Here's how the part is built. I have some questions about the finished solid (model axes, mm). Face numbers are marked on the shaded views. A direction names the side the tool comes from. Coordinates: 2 decimals unless noted, no trailing zeros. Write each loop counter-clockwise with the first axis right and the second up, starting at its lowest first coordinate (ties: lowest second). Pieces come first, ordered by that corner, then holes.
Item 1: I'm going to push flat-ended pins straight in: pin 1 Ø14 at (x, y) = (6, -3.5) entering from +Z; pin 2 Ø6 at (y, z) = (0.5, 7.5) entering from +X; pin 3 Ø1 at (y, z) = (4, 4.5) entering from +X. Where does each tip first touch, or does it pass through?
Item 2: If I drill on line 1 (X direction, y = 0, z = 8.75); line 2 (Y direction, x = 0, z = 1.35); line 3 (X direction, y = -7.5, z = 6.75), over which ranges is the centre line in solid material (lowest first)?
Item 3: For the marked faces 1, 2 and 3, which set-ups out of +Z, -Z, +X, -X, +Y, -Y let a thin tool reach every point of the face, with its end or its side?
Item 4: If we section it at C-C (z = 1.5): Please give me the cut outline in (x, y).
Item 5: If we section it at B-B (x = 0): Please give me the cut outline in (y, z).
Item 6: If we section it at D-D (y = -13): Please give me the cut outline in (x, z), then the cut area to 3 significant figures.
Item 7: If we section it at A-A (y = 0): Please give me the cut outline in (x, z).
Item 8: We'd pull the mould along Y, two halves only. Please class the marked faces 4, 5, 6 and 7: +Y half, -Y half, draft (parallel to the pull), parting line (faces both ways), or undercut.
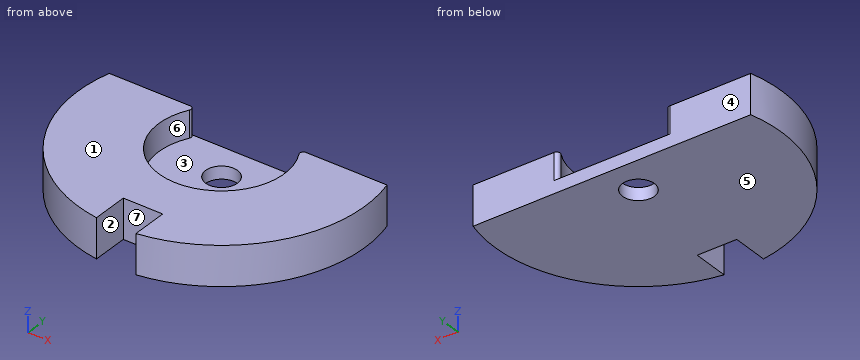
Autodesk Inventor part; units mm, degrees
ref_plane "YZ Plane" through (0, 0, 0) normal (1, 0, 0) x (0, 1, 0)
ref_plane "XZ Plane" through (0, 0, 0) normal (0, 1, 0) x (-1, 0, 0)
ref_plane "XY Plane" through (0, 0, 0) normal (0, 0, 1) x (1, 0, 0)
sketch "Эскиз1" plane through (0, 0, 0) normal (0, 0, 1) x (1, 0, 0)
  line L0 (0, 0) -> (-6, 0) construction
  line L1 (-6, 0) -> (-6, -27.9727) construction
  line L2 (-6, -27.9727) -> (0, -27.9727) construction
  line L3 (0, -27.9727) -> (0, 0) construction
  line L4 (6, -39.5474) -> (6, -29.5474)
  line L5 (6, -29.5474) -> (-6, -29.5474)
  line L6 (-6, -29.5474) -> (-6, -39.5474)
  circle A0 centre (0, 0) radius 4.45
  circle A1 centre (0, 0) radius 40
  line L7 (29.5474, -6) -> (39.5474, -6)
  line L8 (29.5474, 6) -> (29.5474, -6)
  line L9 (39.5474, 6) -> (29.5474, 6)
  line L10 (6, 29.5474) -> (6, 39.5474)
  line L11 (-6, 29.5474) -> (6, 29.5474)
  line L12 (-6, 39.5474) -> (-6, 29.5474)
  line L13 (-29.5474, 6) -> (-39.5474, 6)
  line L14 (-29.5474, -6) -> (-29.5474, 6)
  line L15 (-39.5474, -6) -> (-29.5474, -6)
  line L16 (38.7298, 10) -> (-38.7298, 10)
  circle A2 centre (0, 0) radius 17.5
  line L17 (0, -40) -> (0, -29.6)
  line L18 (0, -29.6) -> (-6, -29.6)
  line L19 (0, -29.6) -> (6, -29.6)
  line L20 (5.5, -29.5474) -> (5.5, -39.6201)
  line L21 (-5.5, -29.5474) -> (-5.5, -39.6201)
  point P0 (6, -34.4819)
  point P1 (6, -27.9727)
  point P2 (6, -39.5474)
  point P3 (6, -39.5474)
  point P4 (-14.3614, 10)
  point P5 (14.3614, 10)
  point P6 (5.5, -29.6)
  point P7 (-5.5, -29.6)
  dimension "d1" = 6
  dimension "d2" = 12
  dimension "d3" = 10
  dimension "d6" = 8.9
  dimension "d12" = 80
  dimension "d15" = 360
  dimension "d19" = 35
  dimension "d24" = 10.4
  dimension "d25" = 0.5
ref_plane "РабПлоскость2" through (0, 0, 0.2) normal (0, 0, 1) x (1, 0, 0)
extrude "Выдавливание4" add sketch "Эскиз1" along normal blind 3.5 contours A2 L16 picked at (-0.1788, 8.1392)
extrude "Выдавливание5" add sketch "Эскиз1" along normal blind 11 contours A1 L20 L19 L4 | L4 L5 L6 A1 L15 L14 L13 L16 A2 L9 L8 L7 | L19 L20 L5 L4 | L7 L8 L9 A1 | A1 L6 L18 L21 | L21 L18 L6 L5 | A1 L13 L14 L15
fillet "Сопряжение1" radius 1 2 edges at (14.3614, 10, 7.25) (-14.3614, 10, 7.25)
properties part number "circle"
Answer list:
1. pin 1: stops at z = 3.5
1. pin 2: stops at x = 40
1. pin 3: stops at x = 39.85
2. line 1: x = -40 to -17.5, 17.5 to 40
2. line 2: y = -29.55 to -4.45, 4.45 to 10
2. line 3: x = -39.29 to -15.81, 15.81 to 39.29
3. face 1: +Z, +X, -X, +Y, -Y
3. face 2: +Z, -Z, -Y
3. face 3: +Z
4. outline: (-38.73, 10) arc R40 ccw to (-5.5, -39.62) - (-5.5, -29.55) - (5.5, -29.55) - (5.5, -39.62) arc R40 ccw to (38.73, 10) - close; hole circle Ø8.9 at (0, 0)
5. outline: (-29.55, 0) - (-4.45, 0) - (-4.45, 3.5) - (-17.5, 3.5) - (-17.5, 11) - (-29.55, 11) - close; (4.45, 0) - (10, 0) - (10, 3.5) - (4.45, 3.5) - close
6. outline: (-37.83, 0) - (37.83, 0) - (37.83, 11) - (11.72, 11) - (11.72, 3.5) - (-11.72, 3.5) - (-11.72, 11) - (-37.83, 11) - close
6. area: 656 mm2
7. outline: (-40, 0) - (-4.45, 0) - (-4.45, 3.5) - (-17.5, 3.5) - (-17.5, 11) - (-40, 11) - close; (4.45, 0) - (40, 0) - (40, 11) - (17.5, 11) - (17.5, 3.5) - (4.45, 3.5) - close
8. face 4: +Y half
8. face 5: draft
8. face 6: undercut
8. face 7: -Y half
